Read the model definition and answer for the solid it produces. Units are mm, in the model's axes. Face numbers are marked on the shaded views. A direction names the side the tool comes from. Give positions to 0.01 mm unless a question says otherwise; leave off trailing zeros. Order: outer loops, then holes, each group sorted by start corner. A loop starts at its lowest first (then second) coordinate and runs counter-clockwise, first axis right, second up. Notation, with made-up numbers: (45, 54) - (87, 54) arc R21 ccw to (87, 89) - close; hole circle Ø2 at (53, 31). An arc over 180 degrees is marked (long way). Use a Markdown table: item, result. Add a question column.
1. A cutting plane is placed at D-D on z = 5.5. Determine the outline of the cut face in (x, y).
2. A cutting plane is placed at A-A on y = 18.5. Determine the outline of the cut face in (x, z), and give its area (3 significant figures).
3. Consider L1, parallel to X at y = 12, z = 16; L2, parallel to X at y = 11, z = 3.5; L3, parallel to Z at x = 14.75, y = 15.5. Determine where each line is inside the solid, lowest interval first.
4. Flat-ended cylindrical pins translate along their axes: P1, Ø3, axis at x = 8, y = 23.5, coming from the +Z side; P2, Ø7, axis at x = 7.5, z = 19.5, coming from the +Y side; P3, Ø5, axis at x = 9, y = 19.5, coming from the -Z side; P4, Ø10, axis at x = 3, z = 14, coming from the +Y side. Find the tip coordinate at first contact, or state that the pin passes through.
5. A cutting plane is placed at C-C on x = 10. Determine the outline of the cut face in (y, z).
6. A cutting plane is placed at B-B on z = 10.75. Determine the outline of the cut face in (x, y).
7. Which of the six approach directions +Z, -Z, +X, -X, +Y, -Y give full straight-line access (tool end or side, diameter ignored) to the marked faces 1, 2, 3, 4 and 5?
8. For a pull along Z with two mould halves and no side action, classify the marked faces 6, 7 and 8 as released by +Z, released by -Z, zero draft, split by the parting line, or undercut.
```python
from build123d import *

# Parameters (mm, degrees)
ESQUISSE1_W                  = 20
ESQUISSE1_H                  = 30
BOSS_EXTRU_1_DEPTH           = 30
COQUE1_START                 = 3
COQUE1_OUTLINE_W             = 25
COQUE1_OUTLINE_H             = 25
COQUE1_DEPTH                 = 14
ENL_V_MAT_EXTRU_1_DEPTH      = 47.904157598
ENL_V_MAT_EXTRU_1_DEPTH_BACK = 47.904157598
ENL_V_MAT_EXTRU_2_DEPTH      = 44.874821937
R_P_TITION_CIRCULAIRE1_COUNT = 2
R_P_TITION_CIRCULAIRE1_ANGLE = 270


# Read off the part's stored shape, not the designer's step: Coque1
with BuildPart() as part:
    # Esquisse1 → Boss.-Extru.1 (new body)
    with BuildSketch(Plane.XY):
        with Locations((10, 15)):
            Rectangle(ESQUISSE1_W, ESQUISSE1_H)
    extrude(amount=BOSS_EXTRU_1_DEPTH)

    # Coque1 outline → Coque1 (cut)
    with BuildSketch(Plane.YZ.offset(COQUE1_START)):
        with Locations((17.5, 17.5)):
            Rectangle(COQUE1_OUTLINE_W, COQUE1_OUTLINE_H)
    extrude(amount=COQUE1_DEPTH, mode=Mode.SUBTRACT)

    # Esquisse3 → Enlèv. mat.-Extru.1 (cut, two sides: drawn at the far end of the back side and taken through both)
    with BuildSketch(Plane(origin=(20, 0, 0), x_dir=(0, 0, -1), z_dir=(1, 0, 0)).offset(-ENL_V_MAT_EXTRU_1_DEPTH_BACK)):
        Polygon((-5, 30), (-30, 30), (-30, 5), align=None)
    extrude(amount=ENL_V_MAT_EXTRU_1_DEPTH + ENL_V_MAT_EXTRU_1_DEPTH_BACK, mode=Mode.SUBTRACT)

    # Esquisse5 → Enlèv. mat.-Extru.2 (cut, symmetric)
    with BuildSketch(Plane.XY.offset(5)):
        with BuildLine():
            Line((12.5525, 25), (12.5525, 10))
            ThreePointArc((12.5525, 10), (10, 7.4475), (7.4475, 10))
            Line((7.4475, 10), (7.4475, 25))
            ThreePointArc((7.4475, 25), (10, 27.5525), (12.5525, 25))
        make_face()
    enl_v_mat_extru_2 = extrude(amount=ENL_V_MAT_EXTRU_2_DEPTH, both=True, mode=Mode.SUBTRACT)

    # Répétition circulaire1: Enlèv. mat.-Extru.2 ×2 about axis
    r_p_tition_circulaire1_axis = Axis((0, 5, 5), (-1, 0, 0))
    for i in range(1, R_P_TITION_CIRCULAIRE1_COUNT):
        add(enl_v_mat_extru_2.rotate(r_p_tition_circulaire1_axis, i * R_P_TITION_CIRCULAIRE1_ANGLE / (R_P_TITION_CIRCULAIRE1_COUNT - 1)), mode=Mode.SUBTRACT)


solid = part.part
```
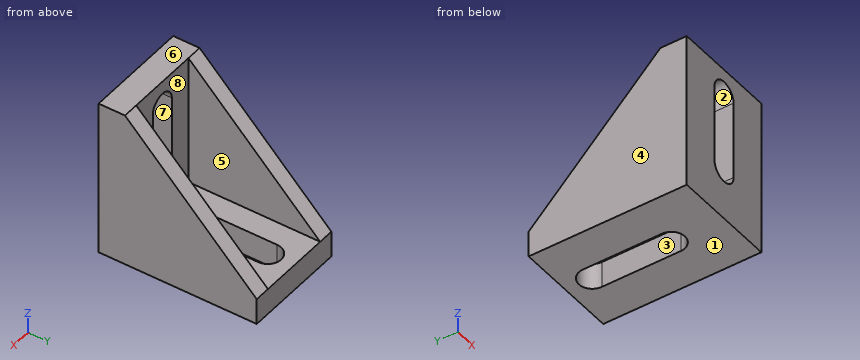
Output values:
| question | item | result |
|---|---|---|
| 1 | outline | (0, 0) - (20, 0) - (20, 29.5) - (17, 29.5) - (17, 5) - (3, 5) - (3, 29.5) - (0, 29.5) - close |
| 2 | outline | (0, 0) - (7.45, 0) - (7.45, 5) - (3, 5) - (3, 16.5) - (0, 16.5) - close; (12.55, 0) - (20, 0) - (20, 16.5) - (17, 16.5) - (17, 5) - (12.55, 5) - close |
| 2 | area | 143 mm² |
| 3 | L1 | 0 to 3, 17 to 20 |
| 3 | L2 | 0 to 7.45, 12.55 to 20 |
| 3 | L3 | 0 to 5 |
| 4 | P1 | z = 5 |
| 4 | P2 | y = 5 |
| 4 | P3 | z = 0 |
| 4 | P4 | y = 26 |
| 5 | outline | (0, 0) - (7.45, 0) - (7.45, 5) - (5, 5) - (5, 7.45) - (0, 7.45) - close; (0, 27.55) - (5, 27.55) - (5, 30) - (0, 30) - close; (27.55, 0) - (30, 0) - (30, 5) - (27.55, 5) - close |
| 6 | outline | (0, 0) - (7.45, 0) - (7.45, 5) - (3, 5) - (3, 24.25) - (0, 24.25) - close; (12.55, 0) - (20, 0) - (20, 24.25) - (17, 24.25) - (17, 5) - (12.55, 5) - close |
| 7 | face 1 | -Z, +X, -X, +Y, -Y |
| 7 | face 2 | +Y, -Y |
| 7 | face 3 | +Z, -Z |
| 7 | face 4 | +Z, -Z, -X, +Y, -Y |
| 7 | face 5 | +Z, +Y |
| 8 | face 6 | released by +Z |
| 8 | face 7 | undercut |
| 8 | face 8 | zero draft |
